Geometry: final body of the model. Coordinates: model frame, mm. A direction names the side the tool comes from. Round coordinates to 2 decimals unless told otherwise and drop trailing zeros. Order: outer loops, then holes, each group sorted by start corner. A loop starts at its lowest first (then second) coordinate and runs counter-clockwise, first axis right, second up. Notation, with made-up numbers: (62, 33) - (90, 33) arc R24 cw to (90, 55) - close; hole circle Ø2 at (4, -37). An arc over 180 degrees is marked (long way). Put each result on its own line as item: value. Start each with the question number.
(1) Section B-B (x = -2). Output: boundary loops of the cut face in (y, z), and give its area (3 significant figures).
(2) Section D-D (z = 0). Output: boundary loops of the cut face in (x, y) (3 decimals), and give its area (3 significant figures).
(3) Pull-direction query (Z, two-part tool) for faces 1 (the face through (-1.5, 0.44, 3.59)), 2 (the face through (-2, 0.889, -3)), 3 (the face through (0.168, 0.438, -5.635)); classes: released by +Z, released by -Z, zero draft, split by the parting line, or undercut.
(4) Pin query (flat end, axial travel): P1, Ø1.1, axis at x = -1.58, z = 4.24, coming from the +Y side. Return the tip coordinate at first contact, or that it passes through.
(5) Access query for faces 4 (the face through (-0.361, 0.4, 4.3)), 5 (the face through (-2.807, 0.4, 4.2)), 6 (the face through (2.807, 0.4, 4.2)), 7 (the face through (1.6, 0.4, 5.462)). Directions: +Z, -Z, +X, -X, +Y, -Y. A direction counts if a zero-diameter tool reaches every point of the face in a straight line with its end or side. Return the directions, or none.
(6) Section C-C (y = 0.3). Output: boundary loops of the cut face in (x, z) (3 decimals), and give its area (3 significant figures).
(7) Section A-A (z = -1.25). Output: boundary loops of the cut face in (x, y), and give its area (3 significant figures).
(8) Material intervals for L1, parallel to Z at x = 1.5, y = 0.5; L2, parallel to X at y = 0.7, z = 3.5; L3, parallel to Z at x = 1.25, y = 0.15, sorted ascending. Write a range as [from, to].
from build123d import *

# Parameters (mm, degrees)
EXTRUDE1_DEPTH     = 0.889
SKETCH5_R          = 0.6604
CUT_EXTRUDE1_DEPTH = 1.889


with BuildPart() as part:
    # Sketch4 → Extrude1 (new body)
    with BuildSketch(Plane(origin=(0, 0, 0), x_dir=(1, 0, 0), z_dir=(0, 1, 0))):
        with BuildLine():
            Line((-2.8067, -5.46211125), (-0.36068, -5.46211125))
            Line((-0.36068, -5.46211125), (-0.36068, -3.154446851))
            ThreePointArc((-0.36068, -3.154446851), (0, 3.175), (0.36068, -3.154446851))
            Line((0.36068, -3.154446851), (0.36068, -5.46211125))
            Line((0.36068, -5.46211125), (2.8067, -5.46211125))
            Line((2.8067, -5.46211125), (2.8067, -2.99831125))
            ThreePointArc((2.8067, -2.99831125), (0, 5.63768875), (-2.8067, -2.99831125))
            Line((-2.8067, -2.99831125), (-2.8067, -5.46211125))
        make_face()
    extrude(amount=EXTRUDE1_DEPTH)

    # Sketch5 → Cut-Extrude1 (cut, through all)
    with BuildSketch(Plane(origin=(0, 0, 0), x_dir=(1, 0, 0), z_dir=(0, 1, 0))):
        with Locations((1.582947052, -4.24322866)):
            Circle(SKETCH5_R)
    cut_extrude1 = extrude(amount=CUT_EXTRUDE1_DEPTH, mode=Mode.SUBTRACT)

    # Mirror1: Cut-Extrude1 across plane
    add(cut_extrude1.mirror(Plane(origin=(0, 0, 0), x_dir=(0, 0, 1), z_dir=(1, 0, 0))), mode=Mode.SUBTRACT)


solid = part.part
Checks:
1. outline: (0, -5.2) - (0.89, -5.2) - (0.89, -2.47) - (0, -2.47) - close; (0, 2.47) - (0.89, 2.47) - (0.89, 3.73) - (0, 3.73) - close; (0, 4.76) - (0.89, 4.76) - (0.89, 5.46) - (0, 5.46) - close
1. area: 4.18 mm²
2. outline: (-4.695, 0) - (-3.175, 0) - (-3.175, 0.889) - (-4.695, 0.889) - close; (3.175, 0) - (4.695, 0) - (4.695, 0.889) - (3.175, 0.889) - close
2. area: 2.70 mm²
3. face 1: undercut
3. face 2: zero draft
3. face 3: split by the parting line
4. P1: passes through
5. face 4: +Z, +Y, -Y
5. face 5: +Z, -X, +Y, -Y
5. face 6: +Z, +X, +Y, -Y
5. face 7: +Z, +X, -X, +Y, -Y
6. outline: (-2.807, 2.998) arc R4.774 ccw (long way) to (2.807, 2.998) - (2.807, 5.462) - (0.361, 5.462) - (0.361, 3.154) arc R3.175 cw (long way) to (-0.361, 3.154) - (-0.361, 5.462) - (-2.807, 5.462) - close; hole circle Ø1.321 at (-1.583, 4.243); hole circle Ø1.321 at (1.583, 4.243)
6. area: 45.9 mm²
7. outline: (-4.76, 0) - (-2.92, 0) - (-2.92, 0.89) - (-4.76, 0.89) - close; (2.92, 0) - (4.76, 0) - (4.76, 0.89) - (2.92, 0.89) - close
7. area: 3.27 mm²
8. L1: z = [-5.4, -2.8], [2.8, 3.59], [4.9, 5.46]
8. L2: x = [-2.81, -0.36], [0.36, 2.81]
8. L3: z = [-5.47, -2.92], [2.92, 3.67], [4.81, 5.46]
